Autodesk Inventor part; units mm, degrees
ref_plane "YZ Plane" through (0, 0, 0) normal (1, 0, 0) x (0, 1, 0)
ref_plane "XZ Plane" through (0, 0, 0) normal (0, 1, 0) x (-1, 0, 0)
ref_plane "XY Plane" through (0, 0, 0) normal (0, 0, 1) x (1, 0, 0)
sketch "Sketch1" plane through (0, 0, 0) normal (0, 0, 1) x (1, 0, 0)
  line L0 (0, 0) -> (82.55, 0)
  line L1 (0, 0) -> (0, 38.1)
  line L2 (0, 38.1) -> (69.85, 38.1)
  line L3 (69.85, 38.1) -> (82.55, 0)
  circle A0 centre (25.4, 19.05) radius 6.35
  dimension "d0" = 82.55
  dimension "d1" = 38.1
  dimension "d2" = 69.85
  dimension "d3" = 12.7
  dimension "d4" = 19.05
  dimension "d5" = 25.4
extrude "Extrusion1" add sketch "Sketch1" along normal blind 19.05
properties part number "final orthograph"
Check sheet for the modelled part. Datum: model origin and axes. Units: mm. Round coordinates to 2 decimals unless told otherwise and drop trailing zeros. Write each loop counter-clockwise with the first axis right and the second up, starting at its lowest first coordinate (ties: lowest second). Pieces come first, ordered by that corner, then holes. Notation, with made-up numbers: M -1.75,68 L 9.25,68 A25 ccw 9.25,81 Z; hole C 42.5,80.5 d3. An arc over 180 degrees is marked long. Write item = value, one per line. Start each with the question number.
1. Release check for a two-part mould opening along X. For faces 1 (the flat face through (41, 0, 9)), 2 (the cylindrical face through (20.36, 22.91, 9.39)), 3 (the flat face through (76.11, 19.32, 9.39)) record: pulls with the +X half, pulls with the -X half, needs draft (parallel to the pull), parting line crosses it, or undercut.
2. Section check D-D, the plane x = 73. Record the cut outline in (y, z), then the cut area to 3 significant figures.
3. Scan lines: line 1 (Y direction, x = 25.4, z = 13.75); line 2 (X direction, y = 21, z = 8.5); line 3 (X direction, y = 2.5, z = 17.25). Record each from-to range of solid material in increasing order. Write a range as [from, to].
4. Section check A-A, the plane x = 25.4. Record the cut outline in (y, z).
5. Section check B-B, the plane z = 6. Record the cut outline in (x, y).
6. Gauge pin test, flat ends, axial feed: pin 1 (4 mm diameter, centred on y = 18.5, z = 6, fed in from +X); pin 2 (1.5 mm diameter, centred on y = 30.5, z = 9, fed in from +X). Record the tip position at first contact, or that the pin passes through.
7. Section check C-C, the plane y = 19.05. Record the cut outline in (x, z), then the cut area to 3 significant figures.
Results found:
q1.face_1 = needs draft
q1.face_2 = undercut
q1.face_3 = pulls with the +X half
q2.outline = M 0,0 L 28.65,0 L 28.65,19.05 L 0,19.05 Z
q2.area = 546 mm^2
q3.line_1 = [0, 12.7], [25.4, 38.1]
q3.line_2 = [0, 19.36], [31.44, 75.55]
q3.line_3 = [0, 81.72]
q4.outline = M 0,0 L 12.7,0 L 12.7,19.05 L 0,19.05 Z; M 25.4,0 L 38.1,0 L 38.1,19.05 L 25.4,19.05 Z
q5.outline = M 0,0 L 82.55,0 L 69.85,38.1 L 0,38.1 Z; hole C 25.4,19.05 d12.7
q6.pin_1 = 77.05
q6.pin_2 = 72.63
q7.outline = M 0,0 L 19.05,0 L 19.05,19.05 L 0,19.05 Z; M 31.75,0 L 76.2,0 L 76.2,19.05 L 31.75,19.05 Z
q7.area = 1,210 mm^2
